The listing builds one solid part. Answer for the finished solid, in the listing's coordinates (mm). A direction names the side the tool comes from. Round coordinates to 2 decimals unless told otherwise and drop trailing zeros. Order: outer loops, then holes, each group sorted by start corner. A loop starts at its lowest first (then second) coordinate and runs counter-clockwise, first axis right, second up. Notation, with made-up numbers: (-38, -28.75) - (-26, -28.75) arc R33 ccw to (-26, 8.25) - close; hole circle Ø11 at (55.25, 45.5). An arc over 180 degrees is marked (long way). Use CSV: the item, a comma, the result in double quotes. Start each with the question number.
Item 1: Straight lines are drawn through the part: line 1 along X through (y, z) = (4.5, -1.5); line 2 along Z through (x, y) = (-8.5, 5); line 3 along Y through (x, z) = (-16, 9). For each, find the intervals that lie inside material, in ascending order. Write a range as [from, to].
Item 2: For faces 4 (the cylindrical face through (-17.43, 4.51, 12.4)), 5 (the flat face through (-20, 4, 0)), determine the directions among +Z, -Z, +X, -X, +Y, -Y from which every point of the face is accessible in a straight line to the end or side of a thin tool.
Item 3: Flat-ended cylindrical pins translate along their axes: P1, Ø6, axis at x = -15.5, z = 7.5, coming from the +Y side; P2, Ø3, axis at y = 1, z = 2, coming from the +X side. Find the tip coordinate at first contact, or state that the pin passes through.
Item 4: Find section A-A, the plane y = 4.5. Give the vertices of the cut face in (x, z).
Item 5: Find section D-D, the plane y = 6.5. Give the vertices of the cut face in (x, z).
Item 6: Determine the mould class of faces 1 (the flat face through (20, 4, 0)), 2 (the cylindrical face through (18.859, 4.465, -13.797)), 3 (the cylindrical face through (0.22, 6.43, 13.6)) for opening direction Z: +Z half, -Z half, draft (parallel to the pull), parting line (faces both ways), or undercut.
```python
from build123d import *

# Parameters (mm, degrees)
BOSS_EXTRU_1_DEPTH      = 7
ENL_V_MAT_EXTRU_1_DEPTH = 5
CONG_1_R                = 2
CONG_2_R                = 2
CONG_3_R                = 2


with BuildPart() as part:
    # Esquisse1 → Boss.-Extru.1 (new body)
    with BuildSketch(Plane(origin=(0, 0, 0), x_dir=(1, 0, 0), z_dir=(0, 1, 0))):
        with BuildLine():
            Line((-16, -15), (16, -15))
            ThreePointArc((16, -15), (18.828427125, -13.828427125), (20, -11))
            Line((20, -11), (20, 11))
            ThreePointArc((20, 11), (18.828427125, 13.828427125), (16, 15))
            Line((16, 15), (-16, 15))
            ThreePointArc((-16, 15), (-18.828427125, 13.828427125), (-20, 11))
            Line((-20, 11), (-20, -11))
            ThreePointArc((-20, -11), (-18.828427125, -13.828427125), (-16, -15))
        make_face()
    extrude(amount=BOSS_EXTRU_1_DEPTH)

    # Esquisse2 → Enlèv. mat.-Extru.1 (cut)
    with BuildSketch(Plane(origin=(0, 7, 0), x_dir=(1, 0, 0), z_dir=(0, 1, 0))):
        with BuildLine():
            Line((18, -11), (18, 11))
            ThreePointArc((18, 11), (17.414213562, 12.414213562), (16, 13))
            Line((16, 13), (-16, 13))
            ThreePointArc((-16, 13), (-17.414213562, 12.414213562), (-18, 11))
            Line((-18, 11), (-18, -11))
            ThreePointArc((-18, -11), (-17.414213562, -12.414213562), (-16, -13))
            Line((-16, -13), (16, -13))
            ThreePointArc((16, -13), (17.414213562, -12.414213562), (18, -11))
        make_face()
    extrude(amount=-ENL_V_MAT_EXTRU_1_DEPTH, mode=Mode.SUBTRACT)

    # Congé1
    cong_1_edges = [part.edges().sort_by_distance(p)[0] for p in [
        (17.414213562, 2, -12.414213562),
        (18, 2, 0),
        (17.414213562, 2, 12.414213562),
        (0, 2, 13),
        (-17.414213562, 2, 12.414213562),
        (-18, 2, 0),
        (-17.414213562, 2, -12.414213562),
        (0, 2, -13),
    ]]
    fillet(cong_1_edges, radius=CONG_1_R)

    # Congé2
    cong_2_edges = [part.edges().sort_by_distance(p)[0] for p in [
        (0, 0, 15),
        (-18.828427125, 0, 13.828427125),
        (-20, 0, 0),
        (-18.828427125, 0, -13.828427125),
        (0, 0, -15),
        (18.828427125, 0, -13.828427125),
        (20, 0, 0),
        (18.828427125, 0, 13.828427125),
    ]]
    fillet(cong_2_edges, radius=CONG_2_R)

    # Congé3
    cong_3_edges = [part.edges().sort_by_distance(p)[0] for p in [
        (17.414213562, 7, -12.414213562),
        (0, 7, -13),
        (-17.414213562, 7, -12.414213562),
        (-18, 7, 0),
        (-17.414213562, 7, 12.414213562),
        (0, 7, 13),
        (17.414213562, 7, 12.414213562),
        (18, 7, 0),
    ]]
    fillet(cong_3_edges, radius=CONG_3_R - 0.0001)  # a hair under: the kernel refuses the full size


solid = part.part
```
Worked out:
1,line 1,"x = [-20, -18], [18, 20]"
1,line 2,"z = [-15, -13], [13, 15]"
1,line 3,"y = [0, 2]"
2,face 4,"+Y"
2,face 5,"+Z, -Z, -X, +Y, -Y"
3,P1,"stops at y = 6.32"
3,P2,"stops at x = 20"
4,outline,"(-20, -11) arc R4 ccw to (-16, -15) - (16, -15) arc R4 ccw to (20, -11) - (20, 11) arc R4 ccw to (16, 15) - (-16, 15) arc R4 ccw to (-20, 11) - close; hole (-18, -11) arc R2 ccw to (-16, -13) - (16, -13) arc R2 ccw to (18, -11) - (18, 11) arc R2 ccw to (16, 13) - (-16, 13) arc R2 ccw to (-18, 11) - close"
5,outline,"(-20, -11) arc R4 ccw to (-16, -15) - (16, -15) arc R4 ccw to (20, -11) - (20, 11) arc R4 ccw to (16, 15) - (-16, 15) arc R4 ccw to (-20, 11) - close; hole (-18.68, -11) arc R2.68 ccw to (-16, -13.68) - (16, -13.68) arc R2.68 ccw to (18.68, -11) - (18.68, 11) arc R2.68 ccw to (16, 13.68) - (-16, 13.68) arc R2.68 ccw to (-18.68, 11) - close"
6,face 1,"draft"
6,face 2,"-Z half"
6,face 3,"undercut"
